from build123d import *

# Parameters (mm, degrees)
SKETCH1_R                        = 18.5
BOSS_EXTRUDE1_DEPTH              = 19
SKETCH4_R                        = 6
BOSS_EXTRUDE4_DEPTH              = 6
CUT_EXTRUDE2_DEPTH               = 1
TALADRO_DE_MARGEN_PARA_M31_D     = 3.4
TALADRO_DE_MARGEN_PARA_M31_DEPTH = 6
TALADRO_DE_MARGEN_PARA_M31_TIP   = 1.021463052
CROQUIS1_R                       = 18
CORTAR_EXTRUIR2_DEPTH            = 12
CORTAR_EXTRUIR3_REACH            = 38.187
CROQUIS2_R                       = 3
CROQUIS3_R                       = 18
SALIENTE_EXTRUIR1_DEPTH          = 0.5
SKETCH11_R                       = 2
CUT_EXTRUDE3_DEPTH               = 10
SKETCH12_W                       = 12.5
SKETCH12_H                       = 1.5
CUT_EXTRUDE4_DEPTH               = 0.15
SKETCH13_R                       = 6
CUT_EXTRUDE5_DEPTH               = 10
SKETCH14_R                       = 2.25
SKETCH14_R_2                     = 2
BOSS_EXTRUDE5_DEPTH              = 1


with BuildPart() as part:
    # Sketch1 → Boss-Extrude1 (new body)
    with BuildSketch(Plane.XY):
        Circle(SKETCH1_R)
    extrude(amount=BOSS_EXTRUDE1_DEPTH)

    # Sketch4 → Boss-Extrude4 (add)
    with BuildSketch(Plane.XY.offset(19)):
        with Locations((0, 7)):
            Circle(SKETCH4_R)
    extrude(amount=BOSS_EXTRUDE4_DEPTH)

    # Sketch8 → Cut-Extrude2 (cut)
    with BuildSketch(Plane.XY.offset(19)):
        with BuildLine():
            ThreePointArc((7.635768375, 9.386428571), (0, -12.1), (-7.635768375, 9.386428571))
            ThreePointArc((-7.635768375, 9.386428571), (0, -1), (7.635768375, 9.386428571))
        make_face()
    extrude(amount=-CUT_EXTRUDE2_DEPTH, mode=Mode.SUBTRACT)

    # Taladro de margen para M31
    with Locations(Plane.XY.offset(19)):
        with Locations((7.65, -13.250188678), (-7.65, -13.250188678), (-15.3, 0), (-7.65, 13.250188678), (15.3, 0), (7.65, 13.250188678)):
            Hole(TALADRO_DE_MARGEN_PARA_M31_D / 2, depth=TALADRO_DE_MARGEN_PARA_M31_DEPTH)
            with Locations((0, 0, -(TALADRO_DE_MARGEN_PARA_M31_DEPTH + TALADRO_DE_MARGEN_PARA_M31_TIP / 2))):  # 118° drill point
                Cone(0, TALADRO_DE_MARGEN_PARA_M31_D / 2, TALADRO_DE_MARGEN_PARA_M31_TIP, mode=Mode.SUBTRACT)

    # Croquis1 → Cortar-Extruir2 (cut)
    with BuildSketch(Plane(origin=(0, 0, 0), x_dir=(-1, 0, 0), z_dir=(0, 0, -1))):
        Circle(CROQUIS1_R)
    extrude(amount=-CORTAR_EXTRUIR2_DEPTH, mode=Mode.SUBTRACT)

    # Croquis2 → Cortar-Extruir3 (cut, up to next)
    with BuildSketch(Plane.XY.offset(25), mode=Mode.PRIVATE) as cortar_extruir3_sk1:
        with Locations((0, 7)):
            Circle(CROQUIS2_R)
    cortar_extruir3_tool1 = extrude(cortar_extruir3_sk1.sketch, amount=-CORTAR_EXTRUIR3_REACH, mode=Mode.PRIVATE) & part.part
    add(cortar_extruir3_tool1.solids().sort_by_distance((0, 7, 25))[0], mode=Mode.SUBTRACT)

    # Croquis3 → Saliente-Extruir1 (add)
    with BuildSketch(Plane(origin=(0, 0, 0), x_dir=(-1, 0, 0), z_dir=(0, 0, -1))):
        Circle(CROQUIS3_R)
    extrude(amount=-SALIENTE_EXTRUIR1_DEPTH)

    # Sketch11 → Cut-Extrude3 (cut)
    with BuildSketch(Plane(origin=(0, 0, 0), x_dir=(-1, 0, 0), z_dir=(0, 0, -1))):
        Circle(SKETCH11_R)
    extrude(amount=-CUT_EXTRUDE3_DEPTH, mode=Mode.SUBTRACT)

    # Sketch12 → Cut-Extrude4 (cut)
    with BuildSketch(Plane(origin=(0, 0, 0), x_dir=(-1, 0, 0), z_dir=(0, 0, -1))):
        with Locations((0, -15)):
            Rectangle(SKETCH12_W, SKETCH12_H)
    extrude(amount=-CUT_EXTRUDE4_DEPTH, mode=Mode.SUBTRACT)

    # Sketch13 → Cut-Extrude5 (cut)
    with BuildSketch(Plane(origin=(0, 0, 0), x_dir=(-1, 0, 0), z_dir=(0, 0, -1))):
        Circle(SKETCH13_R)
    extrude(amount=-CUT_EXTRUDE5_DEPTH, mode=Mode.SUBTRACT)

    # Sketch14 → Boss-Extrude5 (add)
    with BuildSketch(Plane(origin=(0, 0, 12), x_dir=(-1, 0, 0), z_dir=(0, 0, -1))):
        with Locations((0, -5.15)):
            Circle(SKETCH14_R)
        with Locations((0, -5.15)):
            Circle(SKETCH14_R_2, mode=Mode.SUBTRACT)
    extrude(amount=BOSS_EXTRUDE5_DEPTH)


solid = part.part
Here's how the part is built. I have some questions about the finished solid (model axes, mm). A direction names the side the tool comes from. Give positions to 0.01 mm unless a question says otherwise; leave off trailing zeros. Order: outer loops, then holes, each group sorted by start corner. A loop starts at its lowest first (then second) coordinate and runs counter-clockwise, first axis right, second up. Notation, with made-up numbers: (63, 68) -> (109, 68) arc R35 cw to (109, 105) -> close; hole circle Ø4 at (59, 87). An arc over 180 degrees is marked (long way). Use a Markdown table: item, result. Add a question column.
Item 1: For faces 1 (the face through (-3, 7, 19)), 2 (the face through (0, -15, 0.15)), 3 (the face through (0.434, -7.102, 11.507)), which set-ups out of +Z, -Z, +X, -X, +Y, -Y let a thin tool reach every point of the face, with its end or its side?
Item 2: Imagine slicing it at D-D on z = 23.25. Please give me the cut outline in (x, y), plus the area to 3 significant figures.
Item 3: Will these pins go through, and if not, where does the flat tip stop? pin 1 (12 mm diameter, centred on x = -2.5, y = -12.5, fed in from +Z); pin 2 (2 mm diameter, centred on x = 0.5, y = -4, fed in from -Z); pin 3 (3 mm diameter, centred on x = -1, y = -5, fed in from -Z); pin 4 (3 mm diameter, centred on y = 12.5, z = 13, fed in from +X).
Item 4: Imagine slicing it at A-A on z = 3.5. Please give me the cut outline in (x, y), plus the area to 3 significant figures.
Item 5: I need wall thicknesses on line 1 (Z direction, x = 7.5, y = 9.5); line 2 (Z direction, x = -4, y = 9.5); line 3 (Y direction, x = 0, z = 11.7). Which ranges of each line are inside material? Lowest first, please.
Item 6: If we mould it in two halves opening along X, with no side actions, what happens to faces 4 (the face through (0, 0, 19)), 5 (the face through (-4.01, -18.06, 9.37)), 6 (the face through (0, -5, 12))? For each: pulls with the +X half, pulls with the -X half, needs draft (parallel to the pull), parting line crosses it, or undercut.
Item 7: Imagine slicing it at B-B on y = -5.15. Please give me the cut outline in (x, z), plus the area to 3 significant figures.
Item 8: Imagine slicing it at C-C on y = 7. Please give me the cut outline in (x, z), plus the area to 3 significant figures.
Data:
| question | item | result |
|---|---|---|
| 1 | face 1 | +Z |
| 1 | face 2 | -Z |
| 1 | face 3 | none |
| 2 | outline | circle Ø12 at (0, 7); hole circle Ø6 at (0, 7) |
| 2 | area | 84.8 mm² |
| 3 | pin 1 | stops at z = 19 |
| 3 | pin 2 | stops at z = 11 |
| 3 | pin 3 | stops at z = 0 |
| 3 | pin 4 | stops at x = 14.87 |
| 4 | outline | circle Ø37 at (0, 0); hole circle Ø36 at (0, 0) |
| 4 | area | 57.3 mm² |
| 5 | line 1 | z = 0 to 0.5, 12 to 19 |
| 5 | line 2 | z = 0 to 0.5, 12 to 25 |
| 5 | line 3 | y = -18.5 to -18, -7.4 to -7.15, -3.15 to -2.9, 18 to 18.5 |
| 6 | face 4 | needs draft |
| 6 | face 5 | parting line crosses it |
| 6 | face 6 | undercut |
| 7 | outline | (-17.77, 0) -> (-3.08, 0) -> (-3.08, 0.5) -> (-17.25, 0.5) -> (-17.25, 12) -> (-2.25, 12) -> (-2.25, 11) -> (-2, 11) -> (-2, 12) -> (2, 12) -> (2, 11) -> (2.25, 11) -> (2.25, 12) -> (17.25, 12) -> (17.25, 0.5) -> (3.08, 0.5) -> (3.08, 0) -> (17.77, 0) -> (17.77, 19) -> (10.95, 19) -> (10.95, 18) -> (-10.95, 18) -> (-10.95, 19) -> (-17.77, 19) -> close |
| 7 | area | 254 mm² |
| 8 | outline | (-17.12, 0) -> (17.12, 0) -> (17.12, 19) -> (9.87, 19) -> (9.87, 18) -> (8, 18) -> (8, 19) -> (6, 19) -> (6, 25) -> (3, 25) -> (3, 12) -> (16.58, 12) -> (16.58, 0.5) -> (-16.58, 0.5) -> (-16.58, 12) -> (-3, 12) -> (-3, 25) -> (-6, 25) -> (-6, 19) -> (-8, 19) -> (-8, 18) -> (-9.87, 18) -> (-9.87, 19) -> (-17.12, 19) -> close |
| 8 | area | 260 mm² |
